Could you check a few things on this drawing? It's one solid part, dimensions in mm from its lowest x, y, z. Round coordinates to 2 decimals unless told otherwise and drop trailing zeros. Write each loop counter-clockwise with the first axis right and the second up, starting at its lowest first coordinate (ties: lowest second). Pieces come first, ordered by that corner, then holes. Notation, with made-up numbers: M -29.75,74 L 15.25,74 A23 ccw 15.25,112 Z; hole C -39,76 d11. An arc over 180 degrees is marked long. One line per item, written item: value. Start each with the question number.
(1) I want a section at D-D on y = 65.5. Please give me the cut outline in (x, z).
(2) Thinking about a two-plate mould opening in X: for the marked faces 1 and 2, which applies, released by +X, released by -X, zero draft, split by the parting line, or undercut?
(3) I want a section at C-C on z = 6.5. Please give me the cut outline in (x, y).
(4) I want a section at A-A on x = 45. Please give me the cut outline in (y, z).
(5) I want a section at B-B on y = 45. Please give me the cut outline in (x, z).
(6) I'm going to push flat-ended pins straight in: pin 1 Ø4.5 at (x, z) = (44.5, 2) entering from -Y; pin 2 Ø2 at (y, z) = (41, 1.5) entering from -X; pin 3 Ø1.2 at (x, z) = (34, 3) entering from +Y. Where does each tip first touch, or does it pass through?
(7) If I drill on L1, parallel to Y at x = 45, z = 5.4; L2, parallel to X at y = 37, z = 5.25; L3, parallel to Z at x = 45, y = 72, over which ranges is the centre line in solid material (lowest first)?
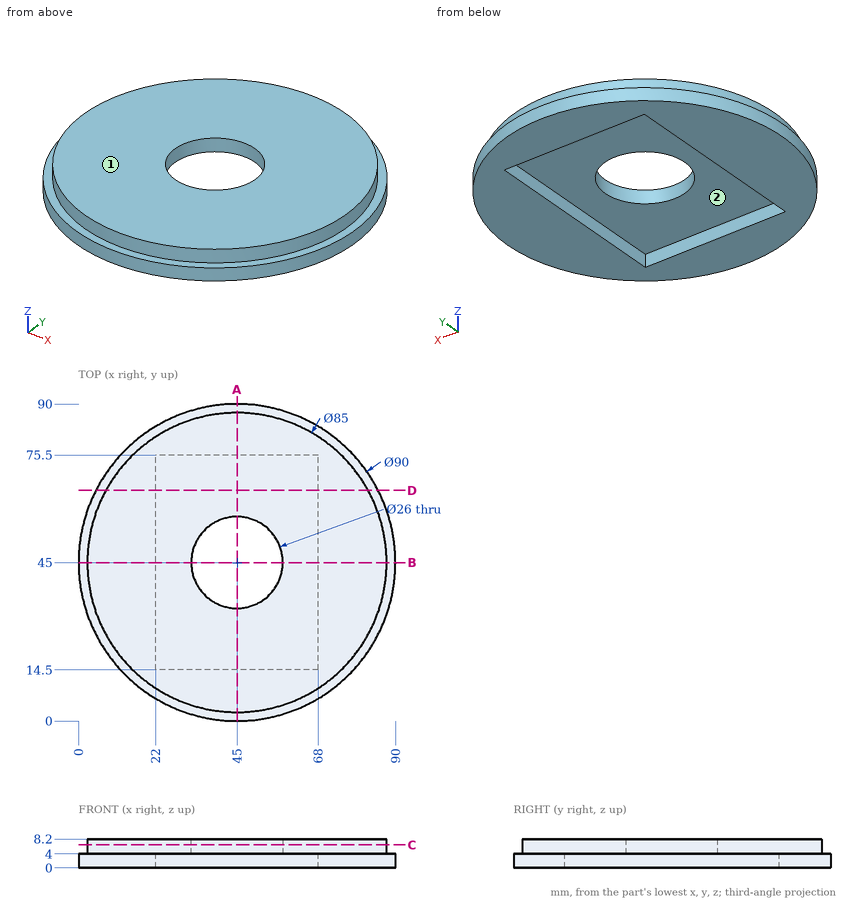
Found:
1. outline: M 4.94,0 L 22,0 L 22,4 L 68,4 L 68,0 L 85.06,0 L 85.06,4 L 82.23,4 L 82.23,8.2 L 7.77,8.2 L 7.77,4 L 4.94,4 Z
2. face 1: zero draft
2. face 2: undercut
3. outline: C 45,45 d85; hole C 45,45 d26
4. outline: M 0,0 L 14.5,0 L 14.5,4 L 32,4 L 32,8.2 L 2.5,8.2 L 2.5,4 L 0,4 Z; M 58,4 L 75.5,4 L 75.5,0 L 90,0 L 90,4 L 87.5,4 L 87.5,8.2 L 58,8.2 Z
5. outline: M 0,0 L 22,0 L 22,4 L 32,4 L 32,8.2 L 2.5,8.2 L 2.5,4 L 0,4 Z; M 58,4 L 68,4 L 68,0 L 90,0 L 90,4 L 87.5,4 L 87.5,8.2 L 58,8.2 Z
6. pin 1: stops at y = 0
6. pin 2: stops at x = 0.1
6. pin 3: stops at y = 88.78
7. L1: y = 2.5 to 32, 58 to 87.5
7. L2: x = 3.26 to 34.75, 55.25 to 86.74
7. L3: z = 4 to 8.2
